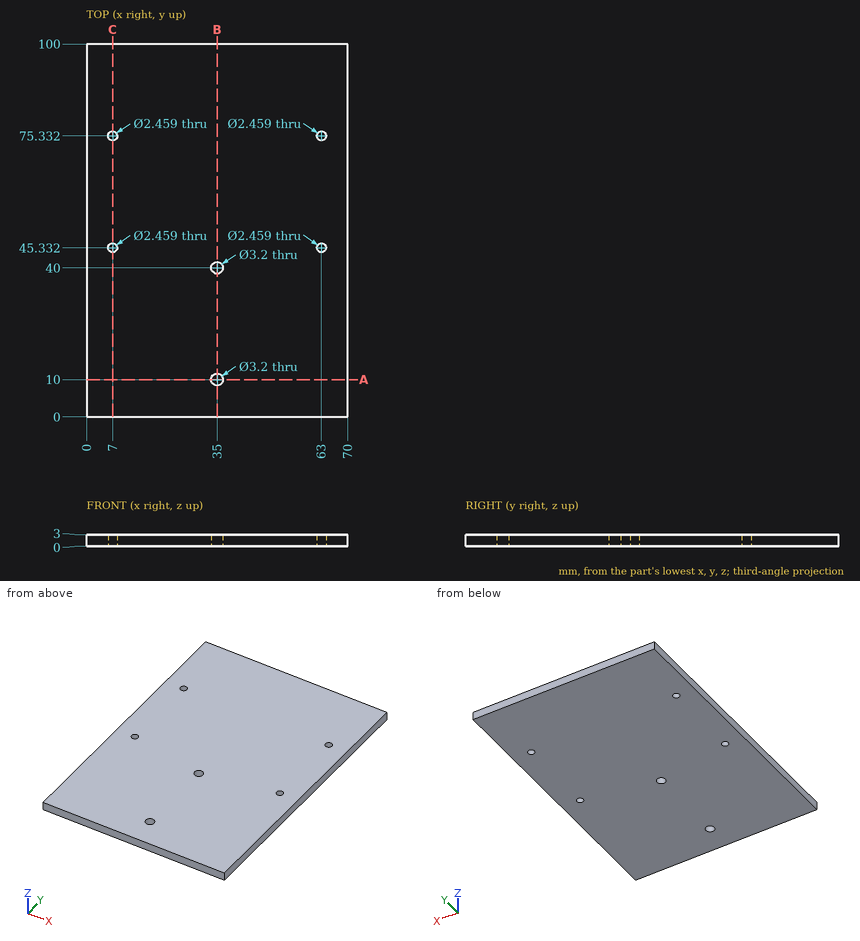
Source: three-view drawing plus pictorial views. Frame: mm from the lowest corner of the part. Coordinates: 2 decimals unless noted, no trailing zeros. Loops run counter-clockwise (first coordinate to the right, second up) from the corner with the lowest first, then second, coordinate; pieces in that order, holes last. Notation, with made-up numbers: (-11.5, -32) - (7.5, -32) arc R16 ccw to (7.5, -26) - close; hole circle Ø6 at (1.5, -0.75). An arc over 180 degrees is marked (long way). Answer in a Markdown table with one row per item. Add a question column.
Item 1: Section query C-C on x = 7. Return the cut outline in (y, z), then the cut area to 3 significant figures.
Item 2: Section query A-A on y = 10. Return the cut outline in (x, z).
Item 3: Line query: line 1 along Y through (x, z) = (35, 0.9); line 2 along Y through (x, z) = (7, 0.95); line 3 along X through (y, z) = (10, 1.1). Output: solid intervals per line, ascending. Write a range as [from, to].
Item 4: Contact query for a flat-ended pin moving along its axis: P1, Ø2.5, axis at x = 35, y = 10, coming from the -Z side. Output: stop coordinate, or through.
Item 5: Section query B-B on x = 35. Return the cut outline in (y, z), then the cut area to 3 significant figures.
Recorded:
| question | item | result |
|---|---|---|
| 1 | outline | (0, 0) - (44.1, 0) - (44.1, 3) - (0, 3) - close; (46.56, 0) - (74.1, 0) - (74.1, 3) - (46.56, 3) - close; (76.56, 0) - (100, 0) - (100, 3) - (76.56, 3) - close |
| 1 | area | 285 mm^2 |
| 2 | outline | (0, 0) - (33.4, 0) - (33.4, 3) - (0, 3) - close; (36.6, 0) - (70, 0) - (70, 3) - (36.6, 3) - close |
| 3 | line 1 | [0, 8.4], [11.6, 38.4], [41.6, 100] |
| 3 | line 2 | [0, 44.1], [46.56, 74.1], [76.56, 100] |
| 3 | line 3 | [0, 33.4], [36.6, 70] |
| 4 | P1 | through |
| 5 | outline | (0, 0) - (8.4, 0) - (8.4, 3) - (0, 3) - close; (11.6, 0) - (38.4, 0) - (38.4, 3) - (11.6, 3) - close; (41.6, 0) - (100, 0) - (100, 3) - (41.6, 3) - close |
| 5 | area | 281 mm^2 |
